The listing builds one solid part. Answer for the finished solid, in the listing's coordinates (mm). Face numbers are marked on the shaded views. A direction names the side the tool comes from. Round coordinates to 2 decimals unless told otherwise and drop trailing zeros. Write each loop counter-clockwise with the first axis right and the second up, starting at its lowest first coordinate (ties: lowest second). Pieces come first, ordered by that corner, then holes. Notation, with made-up numbers: M 6,-22.5 L 65,-22.5 A17 ccw 65,-2.5 Z; hole C 44,51 d2. An arc over 180 degrees is marked long. Put each result on its own line as item: value. Start each with the question number.
```python
from build123d import *

# Parameters (mm, degrees)
SKETCH_W        = 21
SKETCH_H        = 18
PAD_DEPTH       = 7
SKETCH001_W     = 17
SKETCH001_H     = 14
POCKET_DEPTH    = 5
SKETCH003_W     = 17
SKETCH003_H     = 1.5
PAD001_DEPTH    = 1.5
SKETCH004_W     = 1.5
SKETCH004_H     = 11
PAD002_DEPTH    = 1.5
POCKET001_DEPTH = 5
FILLET_R        = 3
SKETCH006_W     = 3.5
SKETCH006_H     = 2.5
POCKET002_DEPTH = 5
SKETCH007_R     = 1.5
PAD003_DEPTH    = 3
SKETCH008_W     = 3
SKETCH008_H     = 7
PAD004_DEPTH    = 10
SKETCH009_R     = 1.6
POCKET003_DEPTH = 15.001
FILLET001_R     = 3
FILLET002_R     = 1


with BuildPart() as part:
    # Sketch → Pad (new body)
    with BuildSketch(Plane.XY):
        with Locations((-10.5, 9)):
            Rectangle(SKETCH_W, SKETCH_H)
    extrude(amount=PAD_DEPTH)

    # Sketch001 (on Face6 of Pad) → Pocket (cut)
    with BuildSketch(Plane.XY.offset(7)):
        with Locations((-10.5, 9)):
            Rectangle(SKETCH001_W, SKETCH001_H)
    extrude(amount=-POCKET_DEPTH, mode=Mode.SUBTRACT)

    # Sketch003 (on Face11 of Pocket) → Pad001 (join)
    with BuildSketch(Plane.XY.offset(2)):
        with Locations((-10.5, 15.25)):
            Rectangle(SKETCH003_W, SKETCH003_H)
        with Locations((-10.5, 2.75)):
            Rectangle(SKETCH003_W, SKETCH003_H)
    extrude(amount=PAD001_DEPTH)

    # Sketch004 (on Face14 of Pad001) → Pad002 (join)
    with BuildSketch(Plane.XY.offset(2)):
        with Locations((-18.25, 9)):
            Rectangle(SKETCH004_W, SKETCH004_H)
        with Locations((-2.75, 9)):
            Rectangle(SKETCH004_W, SKETCH004_H)
    extrude(amount=PAD002_DEPTH)

    # Sketch005 (on Face10 of Pad002) → Pocket001 (cut)
    with BuildSketch(Plane.YZ.offset(-19)):
        with BuildLine():
            ThreePointArc((7, 5.5), (6, 4.5), (7, 3.5))
            Line((7, 3.5), (11, 3.5))
            ThreePointArc((11, 3.5), (12, 4.5), (11, 5.5))
            Line((7, 5.5), (11, 5.5))
        make_face()
    extrude(amount=-POCKET001_DEPTH, mode=Mode.SUBTRACT)

    # Fillet
    fillet_edges = [part.edges().sort_by_distance(p)[0] for p in [
        (0, 0, 3.5),
        (-21, 0, 3.5),
        (-21, 18, 3.5),
        (0, 18, 3.5),
    ]]
    fillet(fillet_edges, radius=FILLET_R)

    # Sketch006 (on Face23 of Pocket001) → Pocket002 (cut)
    with BuildSketch(Plane.XY.offset(2)):
        with Locations((-5.75, 11.75)):
            Rectangle(SKETCH006_W, SKETCH006_H)
    extrude(amount=-POCKET002_DEPTH, mode=Mode.SUBTRACT)

    # Sketch007 (on Face23 of Pocket002) → Pad003 (join)
    with BuildSketch(Plane.XY.offset(2)):
        with Locations((-6.5, 6.5)):
            Circle(SKETCH007_R)
    extrude(amount=PAD003_DEPTH)

    # Sketch008 (on Face7 of Pad003) → Pad004 (join)
    with BuildSketch(Plane(origin=(-21, 0, 0), x_dir=(0, -1, 0), z_dir=(-1, 0, 0))):
        with Locations((-13.5, 3.5)):
            Rectangle(SKETCH008_W, SKETCH008_H)
        with Locations((-4.5, 3.5)):
            Rectangle(SKETCH008_W, SKETCH008_H)
    extrude(amount=PAD004_DEPTH)

    # Sketch009 (on Face17 of Pad004) → Pocket003 (cut, through all)
    with BuildSketch(Plane.XZ.offset(-3)):
        with Locations((-27.429286, 3.5)):
            Circle(SKETCH009_R)
    extrude(amount=-POCKET003_DEPTH, mode=Mode.SUBTRACT)

    # Fillet001
    fillet001_edges = [part.edges().sort_by_distance(p)[0] for p in [
        (-31, 4.5, 7),
        (-31, 4.5, 0),
        (-31, 13.5, 0),
        (-31, 13.5, 7),
    ]]
    fillet(fillet001_edges, radius=FILLET001_R)

    # Fillet002
    fillet002_edges = [part.edges().sort_by_distance(p)[0] for p in [
        (-5.75, 13, 0),
        (-7.5, 11.75, 0),
        (-5.75, 10.5, 0),
        (-4, 11.75, 0),
    ]]
    fillet(fillet002_edges, radius=FILLET002_R)


solid = part.part
```
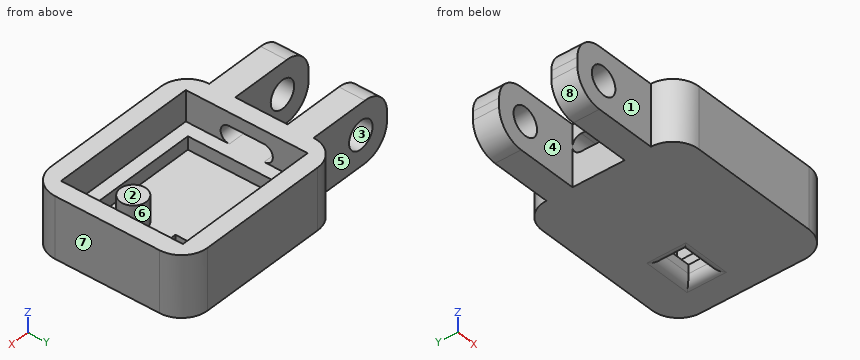
Item 1: Flat-ended cylindrical pins translate along their axes: pin 1 (0.8 mm diameter, centred on y = 11.5, z = 2.5, fed in from -X); pin 2 (1 mm diameter, centred on x = -13.5, y = 12.5, fed in from +Z); pin 3 (5.5 mm diameter, centred on x = -8.5, y = 6.5, fed in from +Z). Find the tip coordinate at first contact, or state that the pin passes through.
Item 2: Section C-C (z = 2.5) is taken. Give the vertices of the cut face in (x, y), and give its area (3 significant figures).
Item 3: Section D-D (z = 6) is taken. Give the vertices of the cut face in (x, y).
Item 4: Section A-A (y = 6.5) is taken. Give the vertices of the cut face in (x, z).
Item 5: Which of the six approach directions +Z, -Z, +X, -X, +Y, -Y give full straight-line access (tool end or side, diameter ignored) to the marked faces 1, 2, 3, 4 and 5?
Item 6: Section B-B (x = -6.5) is taken. Give the vertices of the cut face in (y, z), and give its area (3 significant figures).
Item 7: Consider line 1 along Y through (x, z) = (-7, 6.75); line 2 along Y through (x, z) = (-22, 1.75); line 3 along X through (y, z) = (9.5, 3). Determine where each line is inside the solid, lowest interval first. Write a range as [from, to].
Item 8: Determine the mould class of the marked faces 6, 7 and 8 for opening direction X: released by +X, released by -X, zero draft, split by the parting line, or undercut.
Output values:
1. pin 1: stops at x = -21
1. pin 2: stops at z = 2
1. pin 3: stops at z = 5
2. outline: M -30.96,3 L -28.68,3 L -28.68,6 L -30.96,6 Z; M -30.96,12 L -28.68,12 L -28.68,15 L -30.96,15 Z; M -26.18,3 L -21,3 A3 ccw -18,0 L -3,0 A3 ccw 0,3 L 0,15 A3 ccw -3,18 L -18,18 A3 ccw -21,15 L -26.18,15 L -26.18,12 L -21,12 L -21,6 L -26.18,6 Z; C -6.5,6.5 d3; hole M -17.5,3.5 L -3.5,3.5 L -3.5,14.5 L -17.5,14.5 Z
2. area: 268 mm^2
3. outline: M -30.24,3 L -21,3 A3 ccw -18,0 L -3,0 A3 ccw 0,3 L 0,15 A3 ccw -3,18 L -18,18 A3 ccw -21,15 L -30.24,15 L -30.24,12 L -21,12 L -21,6 L -30.24,6 Z; hole M -19,2 L -2,2 L -2,16 L -19,16 Z
4. outline: M -21,0 L 0,0 L 0,7 L -2,7 L -2,3.5 L -3.5,3.5 L -3.5,2 L -5,2 L -5,5 L -8,5 L -8,2 L -17.5,2 L -17.5,3.5 L -19,3.5 L -19,3.63 L -21,3.63 Z; M -21,5.37 L -19,5.37 L -19,7 L -21,7 Z
5. face 1: +Z, -Z, -X, -Y
5. face 2: +Z
5. face 3: +Y, -Y
5. face 4: +Z, -Z, -X
5. face 5: +Z, -Z, -X, +Y
6. outline: M 0,0 L 9.5,0 A1 ccw 10.5,1 L 10.5,2 L 8,2 L 8,5 L 5,5 L 5,2 L 3.5,2 L 3.5,3.5 L 2,3.5 L 2,7 L 0,7 Z; M 13,1 A1 ccw 14,0 L 18,0 L 18,7 L 16,7 L 16,3.5 L 14.5,3.5 L 14.5,2 L 13,2 Z
6. area: 64.1 mm^2
7. line 1: y = [0, 2], [16, 18]
7. line 2: y = [3, 6], [12, 15]
7. line 3: x = [-21, -17.5], [-3.5, 0]
8. face 6: undercut
8. face 7: released by +X
8. face 8: released by -X
